from build123d import *

# Parameters (mm, degrees)
F6_R      = 12
F4_R      = 24
F7_FACE_R = 24
F5_R      = 24
F8_FACE_R = 24
F3_R      = 22
F10_W     = 12
F10_H     = 3
F11_DEPTH = 10
F12_R     = 6
F13_DEPTH = 3
F14_R     = 2.5
F15_DEPTH = 21.0010001


with BuildPart() as f7:
    # F6 (on offset) → F7 section 0
    with BuildSketch(Plane.XY.offset(-21)):
        Circle(F6_R)
    # F4 (on offset) → F7 section 1
    with BuildSketch(Plane.XY.offset(-4)):
        Circle(F4_R)
    loft()

    # F7_face (on face) → F8 section 0
    with BuildSketch(Plane.XY.offset(-4)):
        Circle(F7_FACE_R)
    # F5 (on Top) → F8 section 1
    with BuildSketch(Plane.XY):
        Circle(F5_R)
    loft()

    # F8_face (on face) → F9 section 0
    with BuildSketch(Plane.XY):
        Circle(F8_FACE_R)
    # F3 (on offset) → F9 section 1
    with BuildSketch(Plane.XY.offset(2)):
        Circle(F3_R)
    loft()

    # F10 (on face) → F11 (join)
    with BuildSketch(Plane(origin=(0, 0, -21), x_dir=(1, 0, 0), z_dir=(0, 0, -1))):
        with Locations((0, -4.5)):
            Rectangle(F10_W, F10_H)
    extrude(amount=F11_DEPTH)

    # F12 (on face) → F13 (join)
    with BuildSketch(Plane.XZ.offset(-3)):
        with Locations((0, -31)):
            Circle(F12_R)
    extrude(amount=-F13_DEPTH)

    # F14 (on face) → F15 (cut, through all)
    with BuildSketch(Plane.XZ.offset(-3)):
        with Locations((0, -31)):
            Circle(F14_R)
    extrude(amount=-F15_DEPTH, mode=Mode.SUBTRACT)

    # F16: F7 across plane


with BuildPart() as f7_1:
    add(f7.part)
    add(f7.part.mirror(Plane.XZ))


solid = f7_1.part
Design review of the part built by this model. Coordinates are the model's own, in mm. A direction names the side the tool comes from. Give positions to 0.01 mm unless a question says otherwise; leave off trailing zeros. Loops run counter-clockwise (first coordinate to the right, second up) from the corner with the lowest first, then second, coordinate; pieces in that order, holes last. Notation, with made-up numbers: (-0.75, -33) - (38.25, -33) arc R20 ccw to (38.25, -11) - close; hole circle Ø6 at (-5.75, -26). An arc over 180 degrees is marked (long way). Use CSV: the item, a comma, the result in double quotes. Start each with the question number.
1. Add section A-A (z = -27). State the section outline as (x, y) points, plus the area to 3 significant figures.
2. Wall thickness on L1, parallel to Z at x = 0, y = 4.35; L2, parallel to Z at x = -5, y = -10; L3, parallel to Y at x = 19, z = -6: over which ranges is each line inside the solid? List them lowest first.
3. Add section B-B (x = 0.5). Count the separate pieces of the cut face and the enclosed holes in it, plus the area to 3 significant figures.
4. Draft analysis for pull direction Y (two halves, no side actions). For faces 6 (the flat face through (0, -3, -27)), 7 (the flat face through (-6, -5, -26)), 8 (the conical face through (-2.764, -12.447, -19.937)), state which applies: released by +Y, released by -Y, zero draft, split by the parting line, or undercut.
5. Insertion check: P1, Ø3, axis at x = 3, z = -16, coming from the -Y side; P2, Ø1.5, axis at y = -9.5, z = -18.5, coming from the -X side; P3, Ø1.5, axis at y = 4.5, z = -16.5, coming from the +X side; P4, Ø19, axis at x = -2, y = -1, coming from the -Z side. Each pin has a flat end and moves straight along its axis. Give the tip position at first contact, or say it passes through.
6. Machinability: for faces 1 (the flat face through (-6, 5, -26)), 2 (the flat face through (0, -6, -27)), 3 (the flat face through (0, 6, -27)), 4 (the flat face through (6, 5, -26)), 5 (the flat face through (0, 3, -27)), which of the approach directions +Z, -Z, +X, -X, +Y, -Y give a long, thin tool a straight path to every point of the face, cutting with its end or side? Answer none if there is none.
7. Add section C-C (z = -17). State the section outline as (x, y) points.
Results found:
1,outline,"(-6, -6) - (6, -6) - (6, -3) - (-6, -3) - close; (-6, 3) - (6, 3) - (6, 6) - (-6, 6) - close"
1,area,"72.0 mm²"
2,L1,"z = -37 to -33.5, -28.5 to 2"
2,L2,"z = -21 to 2"
2,L3,"y = -12.22 to 12.22"
3,separate pieces,"3"
3,enclosed holes,"0"
3,area,"962 mm²"
4,face 6,"undercut"
4,face 7,"zero draft"
4,face 8,"split by the parting line"
5,P1,"stops at y = -16.35"
5,P2,"stops at x = -10.93"
5,P3,"stops at x = 15.09"
5,P4,"stops at z = -37"
6,face 1,"-Z, -X, +Y, -Y"
6,face 2,"-Z, +X, -X, -Y"
6,face 3,"-Z, +X, -X, +Y"
6,face 4,"-Z, +X, +Y, -Y"
6,face 5,"-Z, +X, -X"
7,outline,"circle Ø29.65 at (0, 0)"
